Check sheet for the modelled part. Datum: model origin and axes. Units: mm. Face numbers are marked on the shaded views. A direction names the side the tool comes from. Coordinates: 2 decimals unless noted, no trailing zeros. Write each loop counter-clockwise with the first axis right and the second up, starting at its lowest first coordinate (ties: lowest second). Pieces come first, ordered by that corner, then holes. Notation, with made-up numbers: (42.5, 12.5) -> (66.5, 12.5) arc R13 cw to (66.5, 34.5) -> close; hole circle Ø10 at (60.25, 63). An arc over 180 degrees is marked (long way). Put each result on its own line as item: value.
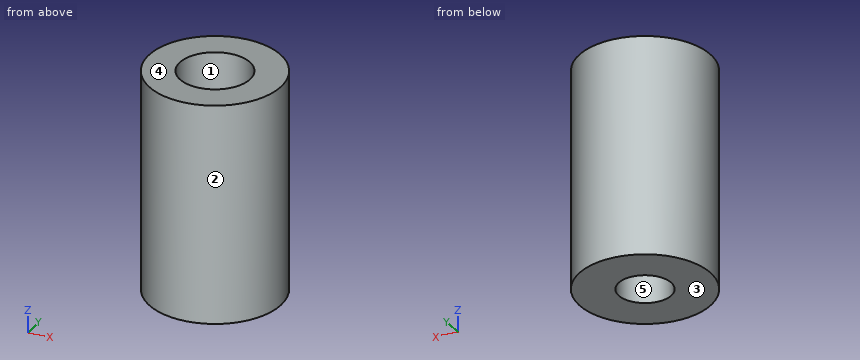
```python
from build123d import *

# Parameters (mm, degrees)
SKETCH_1_R          = 7.5
EXTRUDE_1_DEPTH     = 12.5
SKETCH_2_R          = 3
CUT_EXTRUDE_1_DEPTH = 10
SKETCH_3_R          = 4
CUT_EXTRUDE_2_DEPTH = 9


with BuildPart() as part:
    # 草图1 → 凸台-拉伸1 (new, symmetric)
    with BuildSketch(Plane.XY):
        Circle(SKETCH_1_R)
    extrude(amount=EXTRUDE_1_DEPTH, both=True)

    # 草图2 → 切除-拉伸1 (cut)
    with BuildSketch(Plane(origin=(0, 0, -12.5), x_dir=(-1, 0, 0), z_dir=(0, 0, -1))):
        Circle(SKETCH_2_R)
    extrude(amount=-CUT_EXTRUDE_1_DEPTH, mode=Mode.SUBTRACT)

    # 草图3 → 切除-拉伸2 (cut)
    with BuildSketch(Plane.XY.offset(12.5)):
        Circle(SKETCH_3_R)
    extrude(amount=-CUT_EXTRUDE_2_DEPTH, mode=Mode.SUBTRACT)


solid = part.part
```
Q1. Mould release check, pull along Y, two halves, no side actions. Record for the marked faces 1, 2 and 3: released by +Y, released by -Y, zero draft, split by the parting line, or undercut.
Recorded:
face 1: undercut
face 2: split by the parting line
face 3: zero draft
Q2. Cross-section at D-D (z = -8.75). Record the cut outline in (x, y).
Recorded:
outline: circle Ø15 at (0, 0); hole circle Ø6 at (0, 0)
Q3. Tool access check on the marked faces 4 and 5. Record the directions out of +Z, -Z, +X, -X, +Y, -Y that give a thin tool (end or side, any length) a straight path to the whole face; none if there is none.
Recorded:
face 4: +Z, +X, -X, +Y, -Y
face 5: -Z
Q4. Cross-section at C-C (z = 6.75). Record the cut outline in (x, y), plus the area to 3 significant figures.
Recorded:
outline: circle Ø15 at (0, 0); hole circle Ø8 at (0, 0)
area: 126 mm2
Q5. Material ranges on line 1 along Y through (x, z) = (0, 9.25); line 2 along Y through (x, z) = (0, -8.5); line 3 along Z through (x, y) = (-2, -2.5), recorded low to high.
Recorded:
line 1: y = -7.5 to -4, 4 to 7.5
line 2: y = -7.5 to -3, 3 to 7.5
line 3: z = -12.5 to 3.5
Q6. Depth check by flat-ended pin: P1, Ø8, axis at x = 4.5, z = 7, coming from the -Y side; P2, Ø5, axis at x = 0, y = 0, coming from the -Z side; P3, Ø8, axis at y = -5.5, z = 3, coming from the +X side. Enter the tip coordinate at first touch or a pass-through.
Recorded:
P1: stops at y = -7.48
P2: stops at z = -2.5
P3: stops at x = 7.35
Q7. Cross-section at A-A (y = 0). Record the cut outline in (x, z).
Recorded:
outline: (-7.5, -12.5) -> (-3, -12.5) -> (-3, -2.5) -> (3, -2.5) -> (3, -12.5) -> (7.5, -12.5) -> (7.5, 12.5) -> (4, 12.5) -> (4, 3.5) -> (-4, 3.5) -> (-4, 12.5) -> (-7.5, 12.5) -> close
